```python
from build123d import *

# Parameters (mm, degrees)
SKETCH1_W           = 9.2075
SKETCH1_H           = 7.9375
BOSS_EXTRUDE1_DEPTH = 7.9375
SKETCH2_W           = 5.3975
SKETCH2_H           = 4.953
BOSS_EXTRUDE2_DEPTH = 2.159
SKETCH3_W           = 3.72
SKETCH3_H           = 3.26
CUT_EXTRUDE1_DEPTH  = 1.778
SKETCH4_W           = 9.7155
SKETCH4_H           = 8.4455
SKETCH4_W_2         = 5.3975
SKETCH4_H_2         = 4.953
BOSS_EXTRUDE3_DEPTH = 1.27
BOSS_EXTRUDE4_DEPTH = 0.254
SKETCH7_W           = 3.7
SKETCH7_H           = 3.25
BOSS_EXTRUDE6_DEPTH = 8.72
SKETCH8_W           = 0.5
SKETCH8_H           = 3.25
CUT_EXTRUDE2_DEPTH  = 4
SKETCH6_R           = 0.9525
BOSS_EXTRUDE5_DEPTH = 8.73
SKETCH9_R           = 0.275
BOSS_EXTRUDE7_DEPTH = 2.885


with BuildPart() as part:
    # Sketch1 → Boss-Extrude1 (new body)
    with BuildSketch(Plane(origin=(0, 0, 0), x_dir=(1, 0, 0), z_dir=(0, 1, 0))):
        Rectangle(SKETCH1_W, SKETCH1_H)
    extrude(amount=BOSS_EXTRUDE1_DEPTH)

    # Sketch2 → Boss-Extrude2 (add)
    with BuildSketch(Plane(origin=(0, 7.9375, 0), x_dir=(1, 0, 0), z_dir=(0, 1, 0))):
        Rectangle(SKETCH2_W, SKETCH2_H)
    extrude(amount=BOSS_EXTRUDE2_DEPTH)

    # Sketch3 → Cut-Extrude1 (cut)
    with BuildSketch(Plane(origin=(0, 10.0965, 0), x_dir=(1, 0, 0), z_dir=(0, 1, 0))):
        Rectangle(SKETCH3_W, SKETCH3_H)
    extrude(amount=-CUT_EXTRUDE1_DEPTH, mode=Mode.SUBTRACT)

    # Sketch4 → Boss-Extrude3 (add)
    with BuildSketch(Plane(origin=(0, 7.9375, 0), x_dir=(1, 0, 0), z_dir=(0, 1, 0))):
        Rectangle(SKETCH4_W, SKETCH4_H)
        Rectangle(SKETCH4_W_2, SKETCH4_H_2, mode=Mode.SUBTRACT)
    extrude(amount=-BOSS_EXTRUDE3_DEPTH)

    # Sketch5 → Boss-Extrude4 (add)
    with BuildSketch(Plane(origin=(4.60375, 0, 0), x_dir=(0, 0, -1), z_dir=(1, 0, 0))):
        Polygon((1.524, -0.635), (1.905, 0), (-1.905, 0), (-1.524, -0.635), align=None)
    boss_extrude4 = extrude(amount=-BOSS_EXTRUDE4_DEPTH)

    # Mirror1: Boss-Extrude4 across plane
    add(boss_extrude4.mirror(Plane(origin=(0, 0, 0), x_dir=(0, 0, 1), z_dir=(1, 0, 0))))

    # Sketch7 → Boss-Extrude6 (add)
    with BuildSketch(Plane(origin=(0, 8.3185, 0), x_dir=(1, 0, 0), z_dir=(0, 1, 0))):
        Rectangle(SKETCH7_W, SKETCH7_H)
    extrude(amount=BOSS_EXTRUDE6_DEPTH)

    # Sketch8 → Cut-Extrude2 (cut)
    with BuildSketch(Plane(origin=(0, 17.0385, 0), x_dir=(1, 0, 0), z_dir=(0, 1, 0))):
        with Locations((-1.6, 0)):
            Rectangle(SKETCH8_W, SKETCH8_H)
    extrude(amount=-CUT_EXTRUDE2_DEPTH, mode=Mode.SUBTRACT)

    # Sketch6 → Boss-Extrude5 (add)
    with BuildSketch(Plane(origin=(0, 8.3185, 0), x_dir=(1, 0, 0), z_dir=(0, 1, 0))):
        Circle(SKETCH6_R)
    extrude(amount=BOSS_EXTRUDE5_DEPTH)

    # Sketch9 → Boss-Extrude7 (add)
    with BuildSketch(Plane.XZ):
        with Locations((-2.5, 3)):
            Circle(SKETCH9_R)
        with Locations((2.5, 3)):
            Circle(SKETCH9_R)
        with Locations((2.5, -3)):
            Circle(SKETCH9_R)
        with Locations((-2.5, -3)):
            Circle(SKETCH9_R)
    extrude(amount=BOSS_EXTRUDE7_DEPTH)


solid = part.part
```
The listing builds one solid part. Answer for the finished solid, in the listing's coordinates (mm). A direction names the side the tool comes from. Coordinates: 2 decimals unless noted, no trailing zeros. Write each loop counter-clockwise with the first axis right and the second up, starting at its lowest first coordinate (ties: lowest second). Pieces come first, ordered by that corner, then holes. Notation, with made-up numbers: (22.5, 39) - (28.5, 39) arc R20 cw to (28.5, 46) - close; hole circle Ø8 at (-7, 61.5). An arc over 180 degrees is marked (long way). One line per item, written item: value.
1) Find section D-D (y = 10.75). Give the vertices of the cut face in (x, z) (3 decimals).
Geometry check:
outline: (-1.85, -1.625) - (1.85, -1.625) - (1.85, 1.625) - (-1.85, 1.625) - close
2) Each of these flat-tipped pins is pushed along its axis until it touches: pin 1 Ø1.1 at (x, y) = (0.5, 14.5) entering from -Z (3 decimals); pin 2 Ø1.5 at (x, y) = (3.5, 5.5) entering from +Z; pin 3 Ø1 at (x, z) = (0, -1) entering from +Y; pin 4 Ø4 at (x, y) = (0, 11.5) entering from +Z. Where does it stop, or does it pass through?
Geometry check:
pin 1: stops at z = -1.625
pin 2: stops at z = 3.97
pin 3: stops at y = 17.05
pin 4: stops at z = 2.48
3) Consider line 1 along Y through (x, z) = (-2.75, -1.5); line 2 along Y through (x, z) = (0.25, -0.5); line 3 along X through (y, z) = (5.5, 3.5). Determine where each line is inside the solid, lowest interval first. Write a range as from..to.
Geometry check:
line 1: y = 0..7.94
line 2: y = 0..17.05
line 3: x = -4.6..4.6
4) For a pull along Z with two mould halves and no side action, classify faces 1 (the flat face through (0, 9, 2.476)), 2 (the flat face through (0, 7.938, 3)), 3 (the flat face through (0, 13, 1.625)) as pulls with the +Z half, pulls with the -Z half, needs draft (parallel to the pull), parting line crosses it, or undercut.
Geometry check:
face 1: pulls with the +Z half
face 2: needs draft
face 3: undercut
5) Find section C-C (y = -1.25). Give the vertices of the cut face in (x, z) (3 decimals), and give its area (3 significant figures).
Geometry check:
outline: circle Ø0.55 at (-2.5, -3); circle Ø0.55 at (-2.5, 3); circle Ø0.55 at (2.5, -3); circle Ø0.55 at (2.5, 3)
area: 0.950 mm2
6) A tool of negligible diameter and unlimited length cuts with its end or side. For faces 4 (the flat face through (-1.35, 15, 0)), 5 (the flat face through (0, 3, -3.969)), 6 (the flat face through (2.699, 9, 0)), 7 (the flat face through (4.604, 3, 0)), from which of +Z, -Z, +X, -X, +Y, -Y can it reach the whole face along a straight path? Write none if from no direction.
Geometry check:
face 4: +Z, -Z, -X, +Y
face 5: -Z, +X, -X, -Y
face 6: +Z, -Z, +X, +Y
face 7: +Z, -Z, +X, -Y
